Can you work these out from the model? Positions are in its coordinate system, mm. Give positions to 0.01 mm unless a question says otherwise; leave off trailing zeros. Loops run counter-clockwise (first coordinate to the right, second up) from the corner with the lowest first, then second, coordinate; pieces in that order, holes last. Notation, with made-up numbers: (-15, -5) - (18, -5) arc R29 ccw to (18, 15) - close; hole circle Ø1 at (60.25, 22). An arc over 180 degrees is marked (long way). Use a Markdown table: item, result. Add a question column.
```python
from build123d import *

# Parameters (mm, degrees)
F0_R     = 5.159375
F0_R_2   = 3.571875
F1_DEPTH = 7
F3_DEPTH = 7.001
F4_R     = 0.508


with BuildPart() as f1:
    # F0 (on Top) → F1 (new body)
    with BuildSketch(Plane.XY):
        Circle(F0_R)
        Circle(F0_R_2, mode=Mode.SUBTRACT)
    extrude(amount=F1_DEPTH)

    # F2 (on Top) → F3 (cut, through all)
    with BuildSketch(Plane.XY):
        Polygon((-2.978767, 5.159375), (0, 0), (2.978767, 5.159375), align=None)
    extrude(amount=F3_DEPTH, mode=Mode.SUBTRACT)

    # F4
    f4_edges = [f1.edges().sort_by_distance(p)[0] for p in [
        (1.785938, 3.093334, 3.5),
        (-1.785937, 3.093334, 3.5),
        (-2.579687, 4.46815, 3.5),
        (2.579688, 4.46815, 3.5),
    ]]
    fillet(f4_edges, radius=F4_R)


solid = f1.part
```
1. Suppose I cut it at A-A (y = 0). List the corners of the cut face in (x, z) for me.
2. Will these pins go through, and if not, where does the flat tip stop? P1, Ø1.5, axis at x = 0.5, z = 4.5, coming from the -Y side; P2, Ø2, axis at y = 1.5, z = 6, coming from the -X side; P3, Ø1, axis at y = -4, z = 1.5, coming from the +X side; P4, Ø3, axis at y = -3.5, z = 2, coming from the +X side.
3. Suppose I cut it at D-D (x = 0). List the corners of the cut face in (y, z) for me, and give its area (3 significant figures).
4. Suppose I cut it at C-C (x = -3.25). List the corners of the cut face in (y, z) for me, and give its area (3 significant figures).
5. Suppose I cut it at B-B (z = 5.25). List the corners of the cut face in (x, y) for me, and give its area (3 significant figures).
6. Please list where these lines run through material, in increasing order: line 1 along X through (y, z) = (0, 4); line 2 along Y through (x, z) = (0, 1.5); line 3 along Y through (x, z) = (2.25, 4.25). Write a range as [from, to].
Results below:
| question | item | result |
|---|---|---|
| 1 | outline | (-5.16, 0) - (-3.57, 0) - (-3.57, 7) - (-5.16, 7) - close; (3.57, 0) - (5.16, 0) - (5.16, 7) - (3.57, 7) - close |
| 2 | P1 | y = -5.16 |
| 2 | P2 | x = -5.14 |
| 2 | P3 | x = 3.79 |
| 2 | P4 | x = 4.76 |
| 3 | outline | (-5.16, 0) - (-3.57, 0) - (-3.57, 7) - (-5.16, 7) - close |
| 3 | area | 11.1 mm² |
| 4 | outline | (-4.01, 0) - (-1.48, 0) - (-1.48, 7) - (-4.01, 7) - close; (1.48, 0) - (4.01, 0) - (4.01, 7) - (1.48, 7) - close |
| 4 | area | 35.4 mm² |
| 5 | outline | (-3.05, 4.16) arc R5.16 ccw (long way) to (3.05, 4.16) arc R0.51 ccw to (2.31, 4) - (2.02, 3.51) arc R0.51 ccw to (2.16, 2.85) arc R3.57 cw (long way) to (-2.16, 2.85) arc R0.51 ccw to (-2.02, 3.51) - (-2.31, 4) arc R0.51 ccw to start |
| 5 | area | 36.1 mm² |
| 6 | line 1 | [-5.16, -3.57], [3.57, 5.16] |
| 6 | line 2 | [-5.16, -3.57] |
| 6 | line 3 | [-4.64, -2.77], [2.77, 3.9] |
